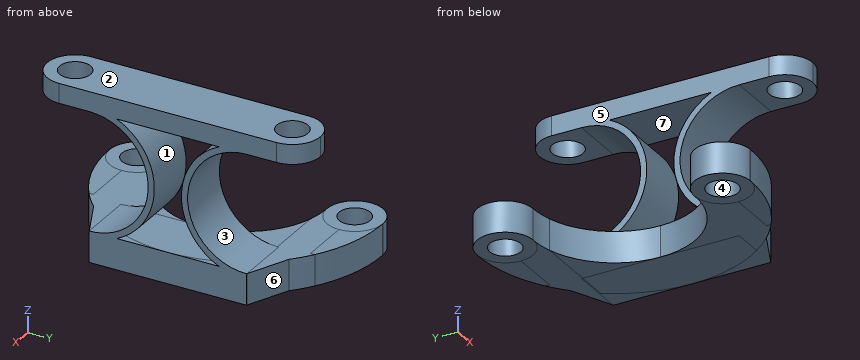
Autodesk Inventor part; units mm, degrees
ref_plane "YZ Plane" through (0, 0, 0) normal (1, 0, 0) x (0, 1, 0)
ref_plane "XZ Plane" through (0, 0, 0) normal (0, 1, 0) x (-1, 0, 0)
ref_plane "XY Plane" through (0, 0, 0) normal (0, 0, 1) x (1, 0, 0)
sketch "Sketch1" plane through (0, 0, 0) normal (0, 0, 1) x (1, 0, 0)
  circle A0 centre (-2.8902, -14) radius 2
  line L0 (-2.8902, -17.5998) -> (-2.8902, -19)
  line L1 (7.1098, -19) -> (-2.8902, -19)
  line L2 (7.1098, -14) -> (7.1098, -19)
  line L3 (7.1098, -14) -> (0.6714, -14)
  arc A1 (0.6714, -14) -> (-2.8902, -10.4002) centre (-2.9286, -14) ccw
  arc A2 (-2.8902, -10.4002) -> (-2.8902, -17.5998) centre (-2.9286, -14) ccw
  circle A3 centre (-2.8902, 14) radius 2
  line L4 (-2.8902, 17.5998) -> (-2.8902, 19)
  arc A4 (-2.8902, 17.5998) -> (-2.8902, 10.4002) centre (-2.9286, 14) ccw
  arc A5 (-2.8902, 10.4002) -> (0.6714, 14) centre (-2.9286, 14) ccw
  line L5 (7.1098, 14) -> (0.6714, 14)
  line L6 (7.1098, 14) -> (7.1098, 19)
  line L7 (7.1098, 19) -> (-2.8902, 19)
  line L8 (9.8002, 10) -> (3.5098, 10)
  line L9 (-57.6094, 10) -> (18.5906, 10)
  arc A6 (-2.8902, -10.4002) -> (-2.8902, 10.4002) centre (-2.7794, 0) ccw
  circle A7 centre (-2.9286, -14) radius 3.6
  circle A8 centre (-2.9286, 14) radius 3.6
  arc A9 (-2.9669, -17.5998) -> (-2.9669, 17.5998) centre (-2.7794, 0) ccw
  point P0 (7.1098, 10)
  point P1 (0, 0)
  point P2 (-2.8902, -17.6004)
  point P3 (-2.8902, 17.6004)
extrude "Extrusion2" add sketch "Sketch1" along normal blind 4 contours A2 A1 A7 | A7 L3 L2 A9 | A1 A6 L9 L8 A9 L2 L3 | L9 L8 A6 A5 L5 L6 A9 | L6 L5 A8 A9 | A4 A8 A5
sketch "Sketch2" plane through (0, 0, 4) normal (0, 0, 1) x (1, 0, 0)
  arc A0 (-2.8902, -17.6004) -> (-2.8902, 17.6004) centre (-2.7794, 0) ccw
  point P0 (0, 0)
  point P1 (14.8214, 0)
ref_plane "Work Plane1" through (14.8214, 0, 4) normal (1, 0, 0) x (0, 1, 0)
sketch "Sketch3" plane through (14.8214, 0, 4) normal (1, 0, 0) x (0, 1, 0)
  line L0 (17.6008, 0) -> (-17.6008, 0)
  arc A0 (-10.16, 0) -> (-10.16, 15.24) centre (-10.16, 7.62) ccw
  line L1 (-10.16, 7.62) -> (-10.16, 0) construction
  line L2 (-10.16, 7.62) -> (-2.54, 7.62) construction
  line L3 (-10.16, 7.62) -> (-10.16, 15.24) construction
  arc A1 (-12.6408, -0.4263) -> (-10.96, 16.0019) centre (-10.16, 7.62) ccw
  line L4 (-10.96, 16.0019) -> (-10.96, 9.0533) construction
  line L5 (0, 0) -> (0, 16.929) construction
  line L6 (-10.16, 15.24) -> (0, 15.24)
  line L7 (-10.16, 15.24) -> (-17.6008, 15.24)
  line L8 (-17.6008, 15.24) -> (-17.6008, 17.78)
  line L9 (-17.6008, 17.78) -> (0, 17.78)
  line L10 (-10.16, 0) -> (-10.16, -0.8)
  line L11 (17.6008, -4) -> (-17.6008, -4)
  line L12 (-10.16, 0) -> (0, 0)
  line L13 (0, 0) -> (0, -4)
  line L14 (0, -4) -> (-10.16, -4)
  line L15 (-10.16, -4) -> (-10.16, 0)
  arc A2 (10.16, 15.24) -> (10.16, 0) centre (10.16, 7.62) ccw
  line L16 (10.16, 7.62) -> (10.16, 0) construction
  line L17 (10.16, 7.62) -> (2.54, 7.62) construction
  line L18 (10.16, 7.62) -> (10.16, 15.24) construction
  arc A3 (10.96, 16.0019) -> (12.6408, -0.4263) centre (10.16, 7.62) ccw
  line L19 (10.96, 16.0019) -> (10.96, 9.0533) construction
  line L20 (10.16, 15.24) -> (0, 15.24)
  line L21 (10.16, 15.24) -> (17.6008, 15.24)
  line L22 (17.6008, 15.24) -> (17.6008, 17.78)
  line L23 (17.6008, 17.78) -> (0, 17.78)
  line L24 (10.16, 0) -> (10.16, -0.8)
  line L25 (10.16, 0) -> (0, 0)
  line L26 (0, -4) -> (10.16, -4)
  line L27 (10.16, -4) -> (10.16, 0)
  point P0 (-17.6004, 0)
  point P1 (17.6004, 0)
  point P2 (-17.6004, -4)
  point P3 (17.6004, -4)
  point P4 (-6.5778, 0)
  point P5 (-6.5778, 15.24)
  point P6 (6.5778, 15.24)
  point P7 (6.5778, 0)
  dimension "d4" = 90
  dimension "d5" = 180
  dimension "d6" = 0.8
  dimension "d7" = 7.62
  dimension "d8" = 10.16
  dimension "d9" = 2.54
extrude "Extrusion3" add sketch "Sketch3" against normal blind 7.2 contours L24 A3 L0 | L0 A3 L20 A2 | A3 L27 L11 L13 L0 | L20 L6 L7 L8 L9 L23 L22 L21 | L13 L11 L15 A1 L0 | A1 L10 L0 | L0 A0 L6 A1
chamfer "Chamfer1" distance 3.175 angle 45 2 edges at (11.5929, -10.16, 2) (11.5929, 10.16, 2)
fillet "Fillet1" radius 3.6 4 edges at (14.8214, -17.6008, 20.51) (14.8214, 17.6008, 20.51) (7.6214, 17.6008, 20.51) (7.6214, -17.6008, 20.51)
sketch "Sketch4" plane through (14.8214, -14.0008, 21.78) normal (0, 0, 1) x (1, 0, 0)
  arc A0 (-7.2, 0) -> (0, 0) centre (-3.6, 0) ccw
  line L0 (0, 28.0016) -> (0, 0)
  arc A1 (0, 28.0016) -> (-7.2, 28.0016) centre (-3.6, 28.0016) ccw
  line L1 (-7.2, 0) -> (-7.2, 28.0016)
  circle A2 centre (-3.6, 0) radius 2
  circle A3 centre (-3.6, 28.0016) radius 2
  point P0 (-14.8214, 14.0008)
  dimension "d16" = 4
  dimension "d17" = 4
hole "Hole1" at (11.2214, -14.0008, 21.78) at (11.2214, 14.0008, 21.78) direction (0, 0, -1) diameter 4 depth 6
properties part number "MotorMountTopSuspension"
CAD build for the part. Positions are in the model's coordinates, mm. Face numbers are marked on the shaded views. A direction names the side the tool comes from. Give positions to 0.01 mm unless a question says otherwise; leave off trailing zeros. Write each loop counter-clockwise with the first axis right and the second up, starting at its lowest first coordinate (ties: lowest second). Pieces come first, ordered by that corner, then holes. Notation, with made-up numbers: M -19,9.25 L -1,9.25 A21 cw -1,34.25 Z; hole C 4.25,-31.75 d1. An arc over 180 degrees is marked long. Put each result on its own line as item: value. Start each with the question number.
(1) Which spindle directions (+Z, -Z, +X, -X, +Y, -Y) get a long thin tool onto all of the face, cutting with end or side? Do the marked faces 5, 6 and 7. Say none if no direction does.
(2) Probe L1, parallel to X at y = -3.5, z = 15.75; L2, parallel to Z at x = 10.5, y = 10; L3, parallel to Z at x = 9.75, y = 2.5. List the from-to ranges inside material, lowest first.
(3) Band-saw the part on D-D, the plane x = 3. Write the cut outline in (y, z), and give its area (3 significant figures).
(4) Band-saw the part on A-A, the plane x = 10.5. Write the cut outline in (y, z).
(5) Band-saw the part on B-B, the plane z = 6. Write the cut outline in (x, y), and give its area (3 significant figures).
(6) Band-saw the part on C-C, the plane y = -4.5. Write the cut outline in (x, z).
(7) Mould opens along Z. For the marked faces 1, 2, 3 and 4 say: +Z half, -Z half, draft (parallel to the pull), parting line (faces both ways), or undercut.
(8) Flat gauge pins, fed straight in: pin 1 Ø3.5 at (x, y) = (-4, -15.5) entering from +Z; pin 2 Ø10 at (x, z) = (7, 18.5) entering from +Y; pin 3 Ø10 at (x, z) = (6, 13.5) entering from -Y; pin 4 Ø3 at (x, z) = (4.5, 4) entering from +Y. Where does each tip first touch, or does it go through?
Response values:
1. face 5: +Z, -X, +Y, -Y
1. face 6: -Z, +X, +Y
1. face 7: +X, -X
2. L1: x = 7.62 to 14.82
2. L2: z = 0 to 4, 19.24 to 21.78
2. L3: z = 0 to 4, 8.12 to 15.12, 19.24 to 21.78
3. outline: M -16.62,0 L -8.65,0 L -8.65,4 L -16.62,4 Z; M 8.65,0 L 16.62,0 L 16.62,4 L 8.65,4 Z
3. area: 63.8 mm2
4. outline: M -17.53,19.24 L -15.87,19.24 L -15.87,21.78 L -17.53,21.78 Z; M -12.14,19.24 L -10.16,19.24 A7.62 cw -10.16,4 L -12.13,4 L -12.13,0 L 12.13,0 L 12.13,4 L 10.16,4 A7.62 cw 10.16,19.24 L 12.14,19.24 L 12.14,21.78 L -12.14,21.78 Z; M 15.87,19.24 L 17.53,19.24 L 17.53,21.78 L 15.87,21.78 Z; hole M -6.58,4 L 6.58,4 A8.42 cw 6.58,19.24 L -6.58,19.24 A8.42 cw Z
5. outline: M 7.62,-5.01 L 14.82,-5.01 L 14.82,-3.89 L 7.62,-3.89 Z; M 7.62,3.89 L 14.82,3.89 L 14.82,5.01 L 7.62,5.01 Z
5. area: 16.2 mm2
6. outline: M 6.6,0 L 14.82,0 L 14.82,4 L 6.6,4 Z; M 7.62,5.39 L 14.82,5.39 L 14.82,6.52 L 7.62,6.52 Z; M 7.62,16.72 L 14.82,16.72 L 14.82,17.85 L 7.62,17.85 Z; M 7.62,19.24 L 14.82,19.24 L 14.82,21.78 L 7.62,21.78 Z
7. face 1: undercut
7. face 2: +Z half
7. face 3: undercut
7. face 4: draft
8. pin 1: stops at z = 4
8. pin 2: stops at y = 17.6
8. pin 3: stops at y = -6.37
8. pin 4: stops at y = 16.62
